```python
from build123d import *

# Parameters (mm, degrees)
F0_R            = 127.5
F0_R_2          = 82.5
F1_DEPTH        = 3
F2_R            = 2.1
F3_DEPTH        = 3
F3_COPIES_COUNT = 6


# Not quite as in the source:
# - a pattern or mirror of a feature is missing from the dataset's text; its kind, count and spacing are read off the source's solid


with BuildPart() as f1:
    # F0 (on Front) → F1 (new body)
    with BuildSketch(Plane.XZ):
        Circle(F0_R)
        Circle(F0_R_2, mode=Mode.SUBTRACT)
    extrude(amount=F1_DEPTH)

    # F2 (on face) → F3 (cut, through all)
    with BuildSketch(Plane.XZ.offset(3)):
        with Locations((0, 97)):
            Circle(F2_R)
    f3 = extrude(amount=-F3_DEPTH, mode=Mode.SUBTRACT)

    # F3_copies: F3 ×6 about axis
    f3_copies_axis = Axis((0, 0, 0), (0, 1, 0))
    for i in range(1, F3_COPIES_COUNT):
        add(f3.rotate(f3_copies_axis, i * 360 / F3_COPIES_COUNT), mode=Mode.SUBTRACT)


solid = f1.part
```
The listing builds one solid part. Answer for the finished solid, in the listing's coordinates (mm). Round coordinates to 2 decimals unless told otherwise and drop trailing zeros. Loops run counter-clockwise (first coordinate to the right, second up) from the corner with the lowest first, then second, coordinate; pieces in that order, holes last. Notation, with made-up numbers: (13.5, 44.25) - (69.5, 44.25) arc R22 cw to (69.5, 75.25) - close; hole circle Ø10 at (3.5, -9). An arc over 180 degrees is marked (long way). Return JSON: item names as keys, results as strings. Group by question number.
1. The part is cut by section B-B on x = -67. Determine the outline of the cut face in (y, z), then the cut area to 3 significant figures.
2. The part is cut by section C-C on y = -1.6. Determine the outline of the cut face in (x, z).
3. The part is cut by section A-A on z = 0. Determine the outline of the cut face in (x, y), then the cut area to 3 significant figures.
4. Each of these flat-tipped pins is pushed along its axis until it touches: P1, Ø4, axis at x = 0, z = -97, coming from the +Y side; P2, Ø1, axis at y = -2.5, z = 87.5, coming from the -X side; P3, Ø10, axis at x = 73, z = -68.5, coming from the +Y side. Where does it stop, or does it pass through?
5. Consider probe 1 along Z at (x, y) = (0, -1.7); probe 2 along Z at (x, y) = (-85, -0.1); probe 3 along X at (y, z) = (-1.5, 97). Determine where each line is inside the solid, lowest interval first.
6. The mould has two halves that part along X. Classify faces 1 (the cylindrical face through (-27.64, -1.48, -124.47)), 2 (the flat face through (-2, 0, -83)), 3 (the cylindrical face through (-17.88, -1.48, -80.54)): pulls with the +X half, pulls with the -X half, needs draft (parallel to the pull), parting line crosses it, or undercut.
7. The part is cut by section D-D on z = 92. Determine the outline of the cut face in (x, y), then the cut area to 3 significant figures.
Resolved:
{
 "1": {"outline": "(-3, -108.48) - (0, -108.48) - (0, -48.14) - (-3, -48.14) - close; (-3, 48.14) - (0, 48.14) - (0, 108.48) - (-3, 108.48) - close", "area": "362 mm²"},
 "2": {"outline": "circle Ø255 at (0, 0); hole circle Ø4.2 at (-84, -48.5); hole circle Ø4.2 at (-84, 48.5); hole circle Ø165 at (0, 0); hole circle Ø4.2 at (0, -97); hole circle Ø4.2 at (0, 97); hole circle Ø4.2 at (84, -48.5); hole circle Ø4.2 at (84, 48.5)"},
 "3": {"outline": "(-127.5, -3) - (-82.5, -3) - (-82.5, 0) - (-127.5, 0) - close; (82.5, -3) - (127.5, -3) - (127.5, 0) - (82.5, 0) - close", "area": "270 mm²"},
 "4": {"P1": "passes through", "P2": "stops at x = -93.21", "P3": "stops at y = 0"},
 "5": {"probe 1": "z = -127.5 to -99.1, -94.9 to -82.5, 82.5 to 94.9, 99.1 to 127.5", "probe 2": "z = -95.03 to -50.35, -46.65 to 46.65, 50.35 to 95.03", "probe 3": "x = -82.75 to -2.1, 2.1 to 82.75"},
 "6": {"face 1": "parting line crosses it", "face 2": "needs draft", "face 3": "undercut"},
 "7": {"outline": "(-88.27, -3) - (88.27, -3) - (88.27, 0) - (-88.27, 0) - close", "area": "530 mm²"}
}
